Autodesk Inventor part; units mm, degrees
ref_plane "YZ Plane" through (0, 0, 0) normal (1, 0, 0) x (0, 1, 0)
ref_plane "XZ Plane" through (0, 0, 0) normal (0, 1, 0) x (-1, 0, 0)
ref_plane "XY Plane" through (0, 0, 0) normal (0, 0, 1) x (1, 0, 0)
sketch "スケッチ1" plane through (0, 0, 0) normal (0, 0, 1) x (1, 0, 0)
  line L0 (0, 0) -> (-26.5, 0)
  line L1 (-26.5, 0) -> (-26.5, 17.5)
  line L2 (-26.5, 17.5) -> (0, 17.5)
  line L3 (0, 17.5) -> (0, 0)
  circle A0 centre (-18.5164, 8.75) radius 3.5
  circle A1 centre (-6.7964, 8.75) radius 3
  dimension "d1" = 26.5
  dimension "d2" = 17.5
  dimension "d3" = 7
  dimension "d4" = 6
  dimension "d5" = 8.75
  dimension "d6" = 8.75
extrude "押し出し1" add sketch "スケッチ1" along normal blind 45 contours L0 L1 L2 L3 | A0 | A1
extrude "押し出し2" add sketch "スケッチ1" against normal blind 3.5 contours A0 | A1
fillet "フィレット1" radius 1 4 edges at (-26.5, 17.5, 22.5) (-26.5, 0, 22.5) (0, 17.5, 22.5) (0, 0, 22.5)
properties part number "Battery06P"
Geometry: final body of the model. Coordinates: model frame, mm. A direction names the side the tool comes from. Coordinates: 2 decimals unless noted, no trailing zeros. Write each loop counter-clockwise with the first axis right and the second up, starting at its lowest first coordinate (ties: lowest second). Pieces come first, ordered by that corner, then holes. Notation, with made-up numbers: (53, -23) - (79, -23) arc R18 cw to (79, 10) - close; hole circle Ø2 at (3.5, 82). An arc over 180 degrees is marked (long way). Return JSON: item names as keys, results as strings.
Item 1: Line query: L1, parallel to Y at x = -18.25, z = -1.5; L2, parallel to Z at x = -4.25, y = 4; L3, parallel to Y at x = -17.25, z = -0.5. Output: solid intervals per line, ascending.
Completed:
{"L1": "y = 5.26 to 12.24", "L2": "z = 0 to 45", "L3": "y = 5.49 to 12.01"}
Item 2: Section query C-C (x = -6.75). Output: boundary loops of the cut face in (y, z), and give its area (3 significant figures).
Completed:
{"outline": "(0, 0) - (5.75, 0) - (5.75, -3.5) - (11.75, -3.5) - (11.75, 0) - (17.5, 0) - (17.5, 45) - (0, 45) - close", "area": "808 mm2"}
Item 3: Section query D-D (y = 11). Output: boundary loops of the cut face in (x, z), and give its area (3 significant figures).
Completed:
{"outline": "(-26.5, 0) - (-21.2, 0) - (-21.2, -3.5) - (-15.84, -3.5) - (-15.84, 0) - (-8.78, 0) - (-8.78, -3.5) - (-4.81, -3.5) - (-4.81, 0) - (0, 0) - (0, 45) - (-26.5, 45) - close", "area": "1,230 mm2"}
Item 4: Section query A-A (y = 8.75). Output: boundary loops of the cut face in (x, z).
Completed:
{"outline": "(-26.5, 0) - (-22.02, 0) - (-22.02, -3.5) - (-15.02, -3.5) - (-15.02, 0) - (-9.8, 0) - (-9.8, -3.5) - (-3.8, -3.5) - (-3.8, 0) - (0, 0) - (0, 45) - (-26.5, 45) - close"}
Item 5: Section query B-B (x = -15.75). Output: boundary loops of the cut face in (y, z), and give its area (3 significant figures).
Completed:
{"outline": "(0, 0) - (6.61, 0) - (6.61, -3.5) - (10.89, -3.5) - (10.89, 0) - (17.5, 0) - (17.5, 45) - (0, 45) - close", "area": "803 mm2"}
Item 6: Pull-direction query (X, two-part tool) for faces 1 (the face through (-15.283, 7.409, -1.726)), 2 (the face through (-26.199, 17.215, 22.815)), 3 (the face through (-4.025, 7.601, -1.726)), 4 (the face through (-13, 9, 45)); classes: +X half, -X half, draft (parallel to the pull), parting line (faces both ways), or undercut.
Completed:
{"face 1": "undercut", "face 2": "-X half", "face 3": "undercut", "face 4": "draft"}
Item 7: Pin query (flat end, axial travel): pin 1 Ø9 at (x, y) = (-13.5, 6.5) entering from -Z; pin 2 Ø2 at (x, y) = (-3, 11) entering from -Z. Return the tip coordinate at first contact, or that it passes through.
Completed:
{"pin 1": "stops at z = -3.5", "pin 2": "stops at z = 0"}
Item 8: Reachability of faces 5 (the face through (-13, 9, 0)), 6 (the face through (0, 9, 22)) from +Z, -Z, +X, -X, +Y, -Y: full face, straight path, thin tool, end or side. Return the list, or none.
Completed:
{"face 5": "-Z", "face 6": "+Z, -Z, +X, +Y, -Y"}
